Geometry check sheet. Reference: the model listing, model coordinates, mm. Coordinates: 2 decimals unless noted, no trailing zeros. Write each loop counter-clockwise with the first axis right and the second up, starting at its lowest first coordinate (ties: lowest second). Pieces come first, ordered by that corner, then holes. Notation, with made-up numbers: (9, -16.75) -> (30, -16.75) arc R32 ccw to (30, 10.25) -> close; hole circle Ø4 at (50, 84.5). An arc over 180 degrees is marked (long way). Answer in a Markdown table with one row per item. Add a question column.
1. Mould release check, pull along X, two halves, no side actions. Record for faces 1 (the flat face through (0, 55, 17)), 2 (the flat face through (26, 55, 17)), 3 (the flat face through (2, 57, 17)): pulls with the +X half, pulls with the -X half, needs draft (parallel to the pull), parting line crosses it, or undercut.
2. Cross-section at A-A on x = 4.75. Record the cut outline in (y, z), and give its area (3 significant figures).
3. Depth check by flat-ended pin: P1, Ø4, axis at x = 9, z = 14, coming from the -Y side. Enter the tip coordinate at first touch or a pass-through.
4. Scan lines: L1, parallel to X at y = 63.75, z = 17.75; L2, parallel to Z at x = 24.5, y = 52.75; L3, parallel to Y at x = 24.5, z = 14.5. Record each from-to range of solid material in increasing order. Write a range as from..to.
```python
from build123d import *

# Parameters (mm, degrees)
F0_R     = 10
F1_DEPTH = 2
F2_R     = 1
F3_DEPTH = 22
F4_R     = 10
F5_DEPTH = 2
F6_R     = 0.99999


# Not quite as in the source:
# - a fillet or chamfer is up to 0.001 mm smaller than in the source, because OpenCascade refuses the exact size


with BuildPart() as f1:
    # F0 (on Right) → F1 (new body)
    with BuildSketch(Plane.YZ):
        with Locations((55.1835894585, 16.7251080275)):
            Circle(F0_R)
    extrude(amount=F1_DEPTH)

    # F2 (on face) → F3 (join)
    with BuildSketch(Plane.YZ.offset(2)):
        with Locations((55.1835894585, 16.7251080275)):
            Circle(F2_R)
    extrude(amount=F3_DEPTH)

    # F4 (on face) → F5 (join)
    with BuildSketch(Plane.YZ.offset(24)):
        with Locations((55.1835894585, 16.7251080275)):
            Circle(F4_R)
    extrude(amount=F5_DEPTH)

    # F6 (radius 1 in the source; OpenCascade refuses exactly that, so slightly less here)
    f6_edges = [f1.edges().sort_by_distance(p)[0] for p in [
        (2, 45.183589, 16.725108),
        (0, 45.183589, 16.725108),
        (26, 45.183589, 16.725108),
        (24, 45.183589, 16.725108),
    ]]
    fillet(f6_edges, radius=F6_R)


solid = f1.part
```
Results found:
| question | item | result |
|---|---|---|
| 1 | face 1 | pulls with the -X half |
| 1 | face 2 | pulls with the +X half |
| 1 | face 3 | undercut |
| 2 | outline | circle Ø2 at (55.18, 16.73) |
| 2 | area | 3.14 mm^2 |
| 3 | P1 | stops at y = 54.49 |
| 4 | L1 | x = 0..2, 24..26 |
| 4 | L2 | z = 7.16..26.29 |
| 4 | L3 | y = 45.57..64.8 |
